The listing builds one solid part. Answer for the finished solid, in the listing's coordinates (mm). Face numbers are marked on the shaded views. Give positions to 0.01 mm unless a question says otherwise; leave off trailing zeros. Order: outer loops, then holes, each group sorted by start corner. A loop starts at its lowest first (then second) coordinate and runs counter-clockwise, first axis right, second up. Notation, with made-up numbers: (11.25, 56.5) -> (38.25, 56.5) arc R23 cw to (38.25, 81.5) -> close; hole circle Ø1 at (85, -15). An arc over 180 degrees is marked (long way). Answer as a JSON object with one key per item and string values. Group by question number.
```python
from build123d import *

# Parameters (mm, degrees)
BOSS_EXTRUDE1_DEPTH = 10


with BuildPart() as part:
    # Sketch1 → Boss-Extrude1 (new, symmetric)
    with BuildSketch(Plane.XY):
        with BuildLine():
            Line((8, 0), (15, 0))
            Line((15, 0), (15, -20))
            Line((15, -20), (-15, -20))
            Line((-15, -20), (-15, 0))
            Line((-15, 0), (-8, 0))
            ThreePointArc((-8, 0), (0, -8), (8, 0))
        make_face()
    extrude(amount=BOSS_EXTRUDE1_DEPTH, both=True)


solid = part.part
```
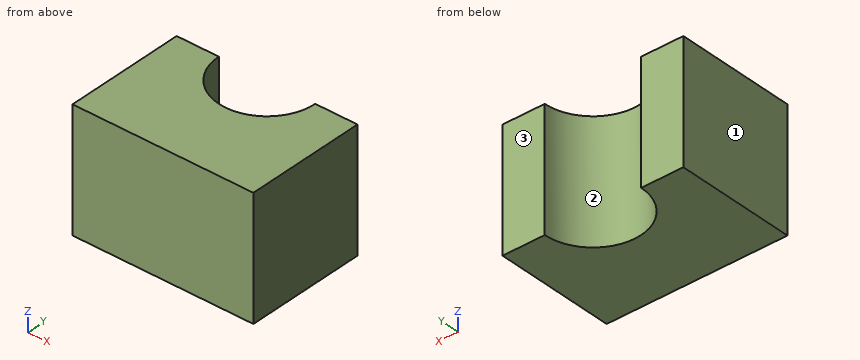
(1) A cutting plane is placed at D-D (x = -6.75). Determine the outline of the cut face in (y, z), and give its area (3 significant figures).
(2) Find the intervals of material crossed by line 1 along X through (y, z) = (-3, -9); line 2 along X through (y, z) = (-4.25, 2.5); line 3 along Y through (x, z) = (5.25, 6.5), in increasing order. Write a range as [from, to].
(3) A flat-ended cylindrical pin translates along its axis: pin 1 Ø5 at (x, z) = (2.5, 5.5) entering from +Y (3 decimals). Find the tip coordinate at first contact, or state that the pin passes through.
(4) A cutting plane is placed at C-C (x = 0). Determine the outline of the cut face in (y, z), and give its area (3 significant figures).
(5) A cutting plane is placed at A-A (y = -6.75). Determine the outline of the cut face in (x, z), and give its area (3 significant figures).
(6) For a pull along X with two mould halves and no side action, classify the marked faces 1, 2 and 3 as +X half, -X half, draft (parallel to the pull), parting line (faces both ways), or undercut.
(7) A cutting plane is placed at B-B (z = 1.25). Determine the outline of the cut face in (x, y).
Check sheet entries:
{
 "1": {"outline": "(-20, -10) -> (-4.29, -10) -> (-4.29, 10) -> (-20, 10) -> close", "area": "314 mm2"},
 "2": {"line 1": "x = [-15, -7.42], [7.42, 15]", "line 2": "x = [-15, -6.78], [6.78, 15]", "line 3": "y = [-20, -6.04]"},
 "3": {"pin 1": "stops at y = -6.245"},
 "4": {"outline": "(-20, -10) -> (-8, -10) -> (-8, 10) -> (-20, 10) -> close", "area": "240 mm2"},
 "5": {"outline": "(-15, -10) -> (-4.29, -10) -> (-4.29, 10) -> (-15, 10) -> close; (4.29, -10) -> (15, -10) -> (15, 10) -> (4.29, 10) -> close", "area": "428 mm2"},
 "6": {"face 1": "-X half", "face 2": "undercut", "face 3": "draft"},
 "7": {"outline": "(-15, -20) -> (15, -20) -> (15, 0) -> (8, 0) arc R8 cw to (-8, 0) -> (-15, 0) -> close"}
}
